Geometry: final body of the model. Coordinates: model frame, mm. Face numbers are marked on the shaded views. A direction names the side the tool comes from. Round coordinates to 2 decimals unless told otherwise and drop trailing zeros. Write each loop counter-clockwise with the first axis right and the second up, starting at its lowest first coordinate (ties: lowest second). Pieces come first, ordered by that corner, then holes.
from build123d import *

# Parameters (mm, degrees)
F1_DEPTH  = 5.5
F2_R      = 1.5
F3_DEPTH  = 25
F5_START  = -0.5
F4_R      = 5.5
F5_DEPTH  = 9
F7_START  = -1.5
F6_W      = 11
F6_H      = 16.464828267
F7_DEPTH  = 3
F8_R      = 1
F9_DEPTH  = 25
F11_DEPTH = 25
F12_R     = 1.2
F13_DEPTH = 7
F14_R     = 1


with BuildPart() as f1:
    # F0 (on Top) → F1 (new body, symmetric)
    with BuildSketch(Plane.XY):
        with BuildLine():
            Line((18, 11), (0, 11))
            ThreePointArc((0, 11), (-11, 0), (0, -11))
            Line((0, -11), (18, -11))
            Line((18, -11), (18, -39))
            Line((18, -39), (23, -39))
            Line((23, -39), (23, 21))
            Line((23, 21), (18, 21))
            Line((18, 21), (18, 11))
        make_face()
    extrude(amount=F1_DEPTH, both=True)

    # F2 (on face) → F3 (cut)
    with BuildSketch(Plane.YZ.offset(23)):
        with Locations((16, 0)):
            Circle(F2_R)
        with Locations((-34, 0)):
            Circle(F2_R)
    extrude(amount=-F3_DEPTH, mode=Mode.SUBTRACT)

    # F4 (on face) → F5 (cut)
    with BuildSketch(Plane.XY.offset(5.5).offset(F5_START)):
        Circle(F4_R)
    extrude(amount=-F5_DEPTH, mode=Mode.SUBTRACT)

    # F6 (on face) → F7 (cut)
    with BuildSketch(Plane(origin=(0, 0, -5.5), x_dir=(1, 0, 0), z_dir=(0, 0, -1)).offset(F7_START)):
        with Locations((0.0076012546, 8.2324141335)):
            Rectangle(F6_W, F6_H)
    extrude(amount=-F7_DEPTH, mode=Mode.SUBTRACT)

    # F8 (on face) → F9 (cut)
    with BuildSketch(Plane.XZ.offset(11)):
        with Locations((0, -2.5)):
            Circle(F8_R)
    extrude(amount=-F9_DEPTH, mode=Mode.SUBTRACT)

    # F10 (on face) → F11 (cut)
    with BuildSketch(Plane.XY.offset(5.5)):
        with BuildLine():
            Line((12, -1), (12, 3))
            ThreePointArc((12, 3), (10.5, 4.5), (9, 3))
            Line((9, 3), (9, -4))
            Line((9, -4), (15, -4))
            Line((15, -4), (15, -11))
            Line((15, -11), (18, -11))
            Line((18, -11), (18, -1))
            Line((18, -1), (12, -1))
        make_face()
    extrude(amount=-F11_DEPTH, mode=Mode.SUBTRACT)

    # F12 (on face) → F13 (cut, through all)
    with BuildSketch(Plane.XZ.offset(11)):
        with Locations((10.5, 0)):
            Circle(F12_R)
    extrude(amount=-F13_DEPTH, mode=Mode.SUBTRACT)

    # F14
    f14_edges = [f1.edges().sort_by_distance(p)[0] for p in [
        (18, 16, 5.5),
        (18, 21, 0),
        (18, 16, -5.5),
        (9, 11, 5.5),
        (18, -20, 5.5),
        (-11, 0, -5.5),
        (7.5, -11, -5.5),
        (18, -20, -5.5),
        (15, -1, -5.5),
        (18, -39, 0),
        (18, -1, 0),
        (12, 1, 5.5),
        (12, -4, 5.5),
        (15, -7.5, -5.5),
        (15, -7.5, 5.5),
        (15, -11, 0),
        (15, -4, 0),
        (12, -1, 0),
        (9, -0.5, -5.5),
        (12, -4, -5.5),
        (9, 11, -5.5),
        (-11, 0, 5.5),
        (7.5, -11, 5.5),
        (9, -0.5, 5.5),
        (10.5, 4.5, 5.5),
        (15, -1, 5.5),
        (10.5, 4.5, -5.5),
    ]]
    fillet(f14_edges, radius=F14_R)


solid = f1.part
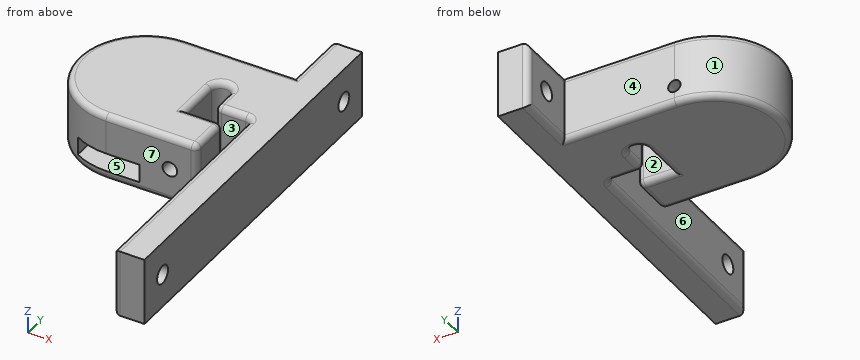
1) Section C-C on y = -34. Output: boundary loops of the cut face in (x, z), plus the area to 3 significant figures.
2) Section B-B on x = 10.5. Output: boundary loops of the cut face in (y, z), plus the area to 3 significant figures.
3) Reachability of the marked faces 5, 6 and 7 from +Z, -Z, +X, -X, +Y, -Y: full face, straight path, thin tool, end or side. Return the list, or none.
4) Section A-A on z = 0. State how many separate pieces and enclosed holes the cut face has, plus the area to 3 significant figures.
5) First-contact query: P1, Ø0.9, axis at y = -3.5, z = -2.5, coming from the -X side; P2, Ø6, axis at x = 9, z = 4, coming from the -Y side; P3, Ø12, axis at x = 2, y = -16.5, coming from the -Z side. Flat tips, straight axial feed; report the tip coordinate or a pass-through.
6) Section D-D on z = 3.75. Output: boundary loops of the cut face in (x, y).
7) Line query: probe 1 along X at (y, z) = (0, 2.25); probe 2 along X at (y, z) = (-3, 0.5); probe 3 along Z at (x, y) = (5, -10). Output: solid intervals per line, ascending.
8) Draft query along Y for the marked faces 1, 2, 3 and 4. Return one class per face: pulls with the +Y half, pulls with the -Y half, needs draft (parallel to the pull), parting line crosses it, or undercut.
Filled in:
1. outline: (18, -4.5) arc R1 ccw to (19, -5.5) - (23, -5.5) - (23, -1.5) - (18, -1.5) - close; (18, 1.5) - (23, 1.5) - (23, 5.5) - (19, 5.5) arc R1 ccw to (18, 4.5) - close
1. area: 39.6 mm2
2. outline: (-11, -4.5) arc R1 ccw to (-10, -5.5) - (-5, -5.5) arc R1 ccw to (-4, -4.5) - (-4, -1.2) - (-11, -1.2) - close; (-11, 1.2) - (-4, 1.2) - (-4, 4.5) arc R1 ccw to (-5, 5.5) - (-10, 5.5) arc R1 ccw to (-11, 4.5) - close; (4.5, -4.5) arc R1 ccw to (5.5, -5.5) - (10, -5.5) arc R1 ccw to (11, -4.5) - (11, 4.5) arc R1 ccw to (10, 5.5) - (5.5, 5.5) arc R1 ccw to (4.5, 4.5) - close
2. area: 130 mm2
3. face 5: -Y
3. face 6: +Z, -Z, -Y
3. face 7: +Z, -Z, -X, -Y
4. separate pieces: 4
4. enclosed holes: 1
4. area: 680 mm2
5. P1: stops at x = -10.57
5. P2: stops at y = -11
5. P3: stops at z = -5.37
6. outline: (0, -11) - (14, -11) arc R1 ccw to (15, -10) - (15, -5) arc R1 ccw to (14, -4) - (9, -4) - (9, 3) arc R1.5 cw to (12, 3) - (12, 0) arc R1 ccw to (13, -1) - (17, -1) arc R1 cw to (18, -2) - (18, -38) arc R1 ccw to (19, -39) - (23, -39) - (23, 21) - (19, 21) arc R1 ccw to (18, 20) - (18, 11) - (0, 11) arc R11 ccw to start; hole circle Ø11 at (0, 0)
7. probe 1: x = -11 to -5.5, 5.5 to 9, 12 to 23
7. probe 2: x = -10.58 to -4.61, 4.61 to 9, 18 to 23
7. probe 3: z = -5.5 to -4, -1 to 5.5
8. face 1: parting line crosses it
8. face 2: undercut
8. face 3: undercut
8. face 4: pulls with the +Y half
